```python
from build123d import *

# Parameters (mm, degrees)
F0_R      = 8
F0_W      = 50
F0_H      = 25
F1_DEPTH  = 30
F0_R_2    = 2
F2_R      = 2.55
F3_DEPTH  = 60
F5_DEPTH  = 30
F6_R      = 4.8374407279
F6_R_2    = 4.05
F7_DEPTH  = 8
F4_R      = 3.025
F8_DEPTH  = 55
F9_DEPTH  = 22
F10_DEPTH = 4
F11_DEPTH = 3
F12_DEPTH = 3
F13_DEPTH = 3
F14_DEPTH = 25
F15_DEPTH = 5
F16_DEPTH = 14.25
F17_DEPTH = 6.25
F19_R     = 3
F20_DEPTH = 50
F22_R     = 4.05
F23_DEPTH = 8


with BuildPart() as f1:
    # F0 (on Front) → F1 (new body)
    with BuildSketch(Plane.XZ):
        with BuildLine():
            Line((-20, 39.2304982366), (-20, 0))
            Line((-20, 0), (140, 0))
            Line((140, 0), (140, 39.3))
            Line((140, 39.3), (129.9754699137, 39.3))
            ThreePointArc((129.9754699137, 39.3), (110, 40), (129.9754699137, 40.7))
            Line((129.9754699137, 40.7), (140, 40.7))
            Line((140, 40.7), (140, 60))
            Line((140, 60), (85, 60))
            Line((85, 60), (85, 55))
            Line((85, 55), (35, 55))
            Line((35, 55), (35, 60))
            Line((35, 60), (-20, 60))
            Line((-20, 60), (-20, 40.7))
            Line((-20, 40.7), (-9.9754699137, 40.7))
            ThreePointArc((-9.9754699137, 40.7), (9.9999392909, 40.0348450672), (-9.9703493939, 39.2304982366))
            Line((-9.9703493939, 39.2304982366), (-20, 39.2304982366))
        make_face()
        with Locations((0, 15)):
            Circle(F0_R, mode=Mode.SUBTRACT)
        with Locations((120, 15)):
            Circle(F0_R, mode=Mode.SUBTRACT)
        with Locations((60, 32.5)):
            Rectangle(F0_W, F0_H, mode=Mode.SUBTRACT)
    extrude(amount=F1_DEPTH)

    # F2 (on Top) → F3 (cut)
    with BuildSketch(Plane.XY):
        with Locations((-13, -15.8086940646)):
            Circle(F2_R)
        with Locations((133, -15.8086940646)):
            Circle(F2_R)
    extrude(amount=F3_DEPTH, mode=Mode.SUBTRACT)

    # F2 (on Top) → F5 (cut)
    with BuildSketch(Plane.XY):
        Polygon((-16.8588337506, -13.5924129261), (-16.8487726432, -18.0424015523), (-12.9899388926, -20.2586826909), (-9.1411662494, -18.0249752032), (-9.1512273568, -13.5749865769), (-13.0100611074, -11.3587054383), align=None)
        with Locations((-13, -15.8086940646)):
            Circle(F2_R, mode=Mode.SUBTRACT)
        Polygon((129.1722717067, -13.5385139461), (129.1201021996, -17.9885139461), (132.9478304928, -20.2586940646), (136.8277282933, -18.0788741831), (136.8798978004, -13.6288741831), (133.0521695072, -11.3586940646), align=None)
        with Locations((133, -15.8086940646)):
            Circle(F2_R, mode=Mode.SUBTRACT)
    extrude(amount=F5_DEPTH, mode=Mode.SUBTRACT)

    # F6 (on Top) → F7 (cut)
    with BuildSketch(Plane.XY):
        with Locations((-13, -15.8086940646)):
            Circle(F6_R)
        with Locations((133, -15.8086940646)):
            Circle(F6_R_2)
    extrude(amount=-F7_DEPTH, mode=Mode.SUBTRACT)

    # F4 (on Top) → F8 (cut)
    with BuildSketch(Plane.XY):
        with Locations((60, -15)):
            Circle(F4_R)
    extrude(amount=-F8_DEPTH, mode=Mode.SUBTRACT)



with BuildPart() as f1b:
    # F0 (on Front) → F1, piece 2 (new body)
    with BuildSketch(Plane.XZ):
        Polygon((-0.0428018717, 19.0412252267), (-3.5212046446, 16.9835451052), (-3.4784027729, 12.9423198784), (0.0428018717, 10.9587747733), (3.5212046446, 13.0164548948), (3.4784027729, 17.0576801216), align=None)
        with Locations((0, 15)):
            Circle(F0_R_2, mode=Mode.SUBTRACT)
    extrude(amount=F1_DEPTH)


with BuildPart() as f1c:
    # F0 (on Front) → F1, piece 3 (new body)
    with BuildSketch(Plane.XZ):
        Polygon((116.4556220174, 17.0463475824), (116.4556220174, 12.9536524176), (120, 10.9073048353), (123.5443779826, 12.9536524176), (123.5443779826, 17.0463475824), (120, 19.0926951647), align=None)
        with Locations((120, 15)):
            Circle(F0_R_2, mode=Mode.SUBTRACT)
    extrude(amount=F1_DEPTH)


with BuildPart() as f1_1:
    add(f1.part)

    add(f1b.part)  # F9 merges F1b

    add(f1c.part)  # F9 merges F1c
    # F0 (on Front) → F9 (join)
    with BuildSketch(Plane.XZ):
        with Locations((0, 15)):
            Circle(F0_R)
        Polygon((-3.4784027729, 12.9423198784), (-3.5212046446, 16.9835451052), (-0.0428018717, 19.0412252267), (3.4784027729, 17.0576801216), (3.5212046446, 13.0164548948), (0.0428018717, 10.9587747733), align=None, mode=Mode.SUBTRACT)
        with Locations((120, 15)):
            Circle(F0_R)
        Polygon((120, 10.9073048353), (116.4556220174, 12.9536524176), (116.4556220174, 17.0463475824), (120, 19.0926951647), (123.5443779826, 17.0463475824), (123.5443779826, 12.9536524176), align=None, mode=Mode.SUBTRACT)
    extrude(amount=F9_DEPTH)

    # F0 (on Front) → F10 (cut)
    with BuildSketch(Plane.XZ):
        Polygon((116.4556220174, 17.0463475824), (116.4556220174, 12.9536524176), (120, 10.9073048353), (123.5443779826, 12.9536524176), (123.5443779826, 17.0463475824), (120, 19.0926951647), align=None)
        with Locations((120, 15)):
            Circle(F0_R_2, mode=Mode.SUBTRACT)
    extrude(amount=-F10_DEPTH, mode=Mode.SUBTRACT)

    # F0 (on Front) → F11 (cut)
    with BuildSketch(Plane.XZ):
        Polygon((116.4556220174, 17.0463475824), (116.4556220174, 12.9536524176), (120, 10.9073048353), (123.5443779826, 12.9536524176), (123.5443779826, 17.0463475824), (120, 19.0926951647), align=None)
        with Locations((120, 15)):
            Circle(F0_R_2, mode=Mode.SUBTRACT)
    extrude(amount=-F11_DEPTH, mode=Mode.SUBTRACT)

    # F0 (on Front) → F12 (cut)
    with BuildSketch(Plane.XZ):
        Polygon((116.4556220174, 17.0463475824), (116.4556220174, 12.9536524176), (120, 10.9073048353), (123.5443779826, 12.9536524176), (123.5443779826, 17.0463475824), (120, 19.0926951647), align=None)
        with Locations((120, 15)):
            Circle(F0_R_2, mode=Mode.SUBTRACT)
    extrude(amount=F12_DEPTH, mode=Mode.SUBTRACT)

    # F0 (on Front) → F13 (cut)
    with BuildSketch(Plane.XZ):
        Polygon((-0.0428018717, 19.0412252267), (-3.5212046446, 16.9835451052), (-3.4784027729, 12.9423198784), (0.0428018717, 10.9587747733), (3.5212046446, 13.0164548948), (3.4784027729, 17.0576801216), align=None)
        with Locations((0, 15)):
            Circle(F0_R_2, mode=Mode.SUBTRACT)
    extrude(amount=F13_DEPTH, mode=Mode.SUBTRACT)

    # F0 (on Front) → F14 (join)
    with BuildSketch(Plane.XZ):
        with Locations((0, 15)):
            Circle(F0_R)
        Polygon((-3.4784027729, 12.9423198784), (-3.5212046446, 16.9835451052), (-0.0428018717, 19.0412252267), (3.4784027729, 17.0576801216), (3.5212046446, 13.0164548948), (0.0428018717, 10.9587747733), align=None, mode=Mode.SUBTRACT)
    extrude(amount=F14_DEPTH)

    # F15 (cut): a face of the model
    f15_faces = [f1_1.faces().sort_by_distance(p)[0] for p in [
        (1.6651859594, -30, 17.9560510216),
    ]]
    extrude(f15_faces, amount=-F15_DEPTH, mode=Mode.SUBTRACT)

    # F16 (cut): a face of the model
    f16_faces = [f1_1.faces().sort_by_distance(p)[0] for p in [
        (116.5639045534, -30, 15),
    ]]
    extrude(f16_faces, amount=-F16_DEPTH, mode=Mode.SUBTRACT)

    # F17 (add, through all): a face of the model
    f17_faces = [f1_1.faces().sort_by_distance(p)[0] for p in [
        (116.5639045534, -15.75, 15),
    ]]
    extrude(f17_faces, amount=F17_DEPTH)

    # F19 (on offset) → F20 (cut)
    with BuildSketch(Plane.XY.offset(55)):
        with Locations((59.9975660443, -15.0059489533)):
            Circle(F19_R)
    extrude(amount=-F20_DEPTH, mode=Mode.SUBTRACT)

    # F22 (on offset) → F23 (cut)
    with BuildSketch(Plane.XY.offset(60)):
        with Locations((-13.0209773779, -15.7698076218)):
            Circle(F22_R)
        with Locations((132.9820901155, -15.7860927284)):
            Circle(F22_R)
    extrude(amount=-F23_DEPTH, mode=Mode.SUBTRACT)


solid = f1_1.part
```
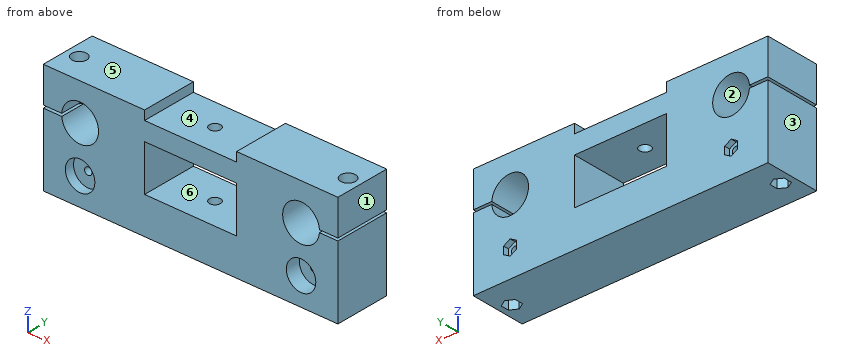
CAD build for the part. Positions are in the model's coordinates, mm. Face numbers are marked on the shaded views. A direction names the side the tool comes from. Round coordinates to 2 decimals unless told otherwise and drop trailing zeros. Order: outer loops, then holes, each group sorted by start corner. A loop starts at its lowest first (then second) coordinate and runs counter-clockwise, first axis right, second up.
Q1. Drop flat-ended pins along their axis: pin 1 (11 mm diameter, centred on x = 133.5, y = -15, fed in from -Z); pin 2 (3 mm diameter, centred on x = 69.5, y = -26.5, fed in from +Z); pin 3 (5 mm diameter, centred on x = -13.5, y = -17, fed in from -Z); pin 4 (3 mm diameter, centred on x = 133, y = -15.81, fed in from +Z). Give the stop position or say it passes through.
Q2. Slice it at B-B (x = 72.5). Write the cut outline in (y, z).
Q3. Slice it at C-C (z = 15). State how many separate pieces and enclosed holes the cut face has, and give its area (3 significant figures).
Q4. Slice it at A-A (y = -23.5). Write the cut outline in (x, z).
Q5. Slice it at D-D (y = -8). Write the cut outline in (x, z).
Q6. Which spindle directions (+Z, -Z, +X, -X, +Y, -Y) get a long thin tool onto all of the face, cutting with end or side? Do the marked faces 4, 5 and 6. Say none if no direction does.
Q7. Wall check: L1, parallel to Z at x = 0, y = -28.7; L2, parallel to Z at x = 120, y = -6.5; L3, parallel to Z at x = 57, y = -10.5. Give the ranges that are in metal, low to high.
Q8. Two-plate mould, pull along X, no slides. Class the marked faces 1, 2 and 3: pulls with the +X half, pulls with the -X half, needs draft (parallel to the pull), parting line crosses it, or undercut.
Results below:
1. pin 1: stops at z = 0
1. pin 2: stops at z = 55
1. pin 3: stops at z = 30
1. pin 4: passes through
2. outline: (-30, 0) - (0, 0) - (0, 20) - (-30, 20) - close; (-30, 45) - (0, 45) - (0, 55) - (-30, 55) - close
3. separate pieces: 3
3. enclosed holes: 3
3. area: 4,250 mm2
4. outline: (-20, 0) - (140, 0) - (140, 39.3) - (129.98, 39.3) arc R10 cw (long way) to (129.98, 40.7) - (140, 40.7) - (140, 60) - (85, 60) - (85, 55) - (35, 55) - (35, 60) - (-20, 60) - (-20, 40.7) - (-9.98, 40.7) arc R10 cw (long way) to (-9.97, 39.23) - (-20, 39.23) - close; hole circle Ø4 at (0, 15); hole (35, 20) - (85, 20) - (85, 45) - (35, 45) - close; hole circle Ø16 at (120, 15)
5. outline: (-20, 0) - (140, 0) - (140, 39.3) - (129.98, 39.3) arc R10 cw (long way) to (129.98, 40.7) - (140, 40.7) - (140, 60) - (85, 60) - (85, 55) - (35, 55) - (35, 60) - (-20, 60) - (-20, 40.7) - (-9.98, 40.7) arc R10 cw (long way) to (-9.97, 39.23) - (-20, 39.23) - close; hole circle Ø4 at (0, 15); hole (35, 20) - (85, 20) - (85, 45) - (35, 45) - close; hole circle Ø4 at (120, 15)
6. face 4: +Z, +Y, -Y
6. face 5: +Z, +X, -X, +Y, -Y
6. face 6: +Y, -Y
7. L1: z = 0 to 7, 23 to 30, 50 to 60
7. L2: z = 0 to 13, 17 to 30, 50 to 60
7. L3: z = 0 to 20, 45 to 55
8. face 1: pulls with the +X half
8. face 2: undercut
8. face 3: pulls with the -X half
